The model under review builds one solid part; all positions refer to its coordinate system, in mm. A direction names the side the tool comes from. Give positions to 0.01 mm unless a question says otherwise; leave off trailing zeros. Order: outer loops, then holes, each group sorted by start corner. A loop starts at its lowest first (then second) coordinate and runs counter-clockwise, first axis right, second up. Notation, with made-up numbers: M 74,27 L 82,27 A24 cw 82,63 Z; hole C -34,46.25 d7. An arc over 180 degrees is marked long. One line per question, with ' | ' between items. Start each with the question number.
1. We need section B-B on y = 19.5. Count the separate pieces of the cut face and the enclosed holes in it, then the cut area to 3 significant figures.
2. Insertion check: P1, Ø10, axis at y = 11.5, z = 34, coming from the +X side; P2, Ø4, axis at x = -39.74, z = 25.77, coming from the +Y side; P3, Ø3, axis at x = -41.46, z = 29.75, coming from the -Y side; P4, Ø2, axis at y = 15.5, z = 11.5, coming from the -X side. Each pin has a flat end and moves straight along its axis. Give the tip position at first contact, or say it passes through.
3. The part is to be moulded in two halves that separate along X. For faces 1 (the face through (-61.67, 12.52, 37.13)), 2 (the face through (-51.286, 18.961, 19.704)), 3 (the face through (-48, 7.62, 27)), 4 (the face through (-44, 25.4, 25)), say which applies: +X half, -X half, draft (parallel to the pull), parting line (faces both ways), or undercut.
4. For faces 5 (the face through (-45.316, 31.661, 26.641)), 6 (the face through (-57.14, 6.26, 24.68)), 7 (the face through (-54.54, 18.96, 25.76)), list the 3-axis set-ups (+Z, -Z, +X, -X, +Y, -Y) from which the entire face can be reached by the end or side of a thin tool; tool diameter is ignored.
5. Wall thickness on L1, parallel to X at y = 17, z = 32; L2, parallel to Y at x = -48, z = 32.5; L3, parallel to Y at x = -47.5, z = 36: over which ranges is each line inside the solid? List them lowest first.
6. We need section D-D on z = 12.5. Write out the cut boundary in (x, y).
7. We need section C-C on x = -37. Write out the cut boundary in (y, z), then the cut area to 3 significant figures.
8. We need section A-A on y = 9. Write out the cut boundary in (x, z) (3 decimals).
```python
from build123d import *

# Parameters (mm, degrees)
F0_R      = 19.05
F1_DEPTH  = 25.4
F2_R      = 9.525
F3_DEPTH  = 12.7
F4_R      = 1.133132
F4_R_2    = 0.889661
F4_R_3    = 0.83878
F4_R_4    = 0.750228
F4_R_5    = 1.060981
F4_R_6    = 1.482769
F4_R_7    = 0.806713
F4_R_8    = 1.482771
F4_R_9    = 1.186214
F4_R_10   = 1.22272
F5_DEPTH  = 25.4
F7_R      = 1.677648
F8_DEPTH  = 5.08
F9_R      = 2.09708
F10_DEPTH = 12.7


with BuildPart() as f1:
    # F0 (on Front) → F1 (new body)
    with BuildSketch(Plane.XZ):
        with Locations((-47.624998, 24.257001)):
            Circle(F0_R)
    extrude(amount=-F1_DEPTH)

    # F2 (on face) → F3 (cut)
    with BuildSketch(Plane.XZ):
        with Locations((-47.624998, 24.257001)):
            Circle(F2_R)
    extrude(amount=-F3_DEPTH, mode=Mode.SUBTRACT)

    # F4 (on face) → F5 (cut)
    with BuildSketch(Plane.XZ.offset(-12.7)):
        with Locations((-41.461259, 29.747711)):
            Circle(F4_R)
        with Locations((-45.970432, 32.532789)):
            Circle(F4_R_2)
        with Locations((-51.010098, 31.604432)):
            Circle(F4_R_3)
        with Locations((-54.060422, 29.482467)):
            Circle(F4_R_4)
        with Locations((-55.519272, 26.166897)):
            Circle(F4_R_5)
        with Locations((-54.193046, 21.5251)):
            Circle(F4_R_6)
        with Locations((-50.479606, 19.668382)):
            Circle(F4_R_7)
        with Locations((-46.103057, 18.6074)):
            Circle(F4_R_8)
        with Locations((-41.461259, 19.933628)):
            Circle(F4_R_9)
        with Locations((-39.737161, 25.769029)):
            Circle(F4_R_10)
    extrude(amount=-F5_DEPTH, mode=Mode.SUBTRACT)

    # F7 (on face) → F8 (join)
    with BuildSketch(Plane.XZ.offset(-12.7)):
        with Locations((-48.044514, 26.577691)):
            Circle(F7_R)
    extrude(amount=F8_DEPTH)

    # F9 (on face) → F10 (join)
    with BuildSketch(Plane(origin=(0, 25.4, 0), x_dir=(-1, 0, 0), z_dir=(0, 1, 0))):
        with Locations((47.411542, 26.54841)):
            Circle(F9_R)
    extrude(amount=F10_DEPTH)


solid = f1.part
```
Entries:
1) separate pieces: 1 | enclosed holes: 10 | area: 1,100 mm^2
2) P1: stops at x = -29.17 | P2: stops at y = 25.4 | P3: stops at y = 0 | P4: stops at x = -62.61
3) face 1: parting line | face 2: undercut | face 3: undercut | face 4: draft
4) face 5: +Y | face 6: -Y | face 7: +Y, -Y
5) L1: x = -65.03 to -51.75, -50.27 to -46.68, -45.26 to -30.22 | L2: y = 12.7 to 25.4 | L3: y = 0 to 25.4
6) outline: M -62.61,0 L -32.64,0 L -32.64,25.4 L -62.61,25.4 Z
7) outline: M 0,8.45 L 25.4,8.45 L 25.4,40.07 L 0,40.07 Z | area: 803 mm^2
8) outline: C -47.625,24.257 d38.1; C -48.045,26.578 d3.355; hole C -47.625,24.257 d19.05
